```python
from build123d import *

# Parameters (mm, degrees)
SKETCH2_R           = 12.5
SKETCH2_R_2         = 15
BOSS_EXTRUDE1_DEPTH = 5


with BuildPart() as part:
    # Sketch2 → Boss-Extrude1 (new body)
    with BuildSketch(Plane.XY):
        with BuildLine():
            ThreePointArc((0, 25), (-25, 0), (0, -25))
            ThreePointArc((0, -25), (28.284271247, -36.715728753), (40, -65))
            ThreePointArc((40, -65), (55.168868326, -87.985840207), (82.267908001, -83.078145737))
            ThreePointArc((82.267908001, -83.078145737), (117.800748333, 0), (82.267908001, 83.078145737))
            ThreePointArc((82.267908001, 83.078145737), (55.168868326, 87.985840207), (40, 65))
            ThreePointArc((40, 65), (28.284271247, 36.715728753), (0, 25))
        make_face()
        Circle(SKETCH2_R, mode=Mode.SUBTRACT)
        with Locations((65, 65)):
            Circle(SKETCH2_R, mode=Mode.SUBTRACT)
        with Locations((65, -65)):
            Circle(SKETCH2_R_2, mode=Mode.SUBTRACT)
        Polygon((75.334929147, -6.098298085), (75.448745635, 5.901162145), (65.113816488, 11.99946023), (54.665070853, 6.098298085), (54.551254365, -5.901162145), (64.886183512, -11.99946023), align=None, mode=Mode.SUBTRACT)
    extrude(amount=BOSS_EXTRUDE1_DEPTH)


solid = part.part
```
Design review of the part built by this model. Coordinates are the model's own, in mm. A direction names the side the tool comes from. Give positions to 0.01 mm unless a question says otherwise; leave off trailing zeros. Write each loop counter-clockwise with the first axis right and the second up, starting at its lowest first coordinate (ties: lowest second). Pieces come first, ordered by that corner, then holes. Notation, with made-up numbers: (67, 41) -> (87, 41) arc R22 cw to (87, 59) -> close; hole circle Ø7 at (16, -6). An arc over 180 degrees is marked (long way). Answer in a Markdown table with one row per item.
(1) For faces 5 (the cylindrical face through (117.793, -1.3, 2.465)), 6 (the flat face through (70.35, 8.91, 2.46)), list the 3-axis set-ups (+Z, -Z, +X, -X, +Y, -Y) from which the entire face can be reached by the end or side of a thin tool; tool diameter is ignored.
Results:
| item | result |
|---|---|
| face 5 | +Z, -Z, +X |
| face 6 | +Z, -Z |
(2) Mouldability with a two-part tool opening along Y and no side actions: class faces 1 (the cylindrical face through (27.972, -36.406, 2.465)), 2 (the cylindrical face through (28.594, 37.028, 2.465)), 3 (the cylindrical face through (55.79, 73.45, 2.46)), 4 (the flat face through (77, 1, 5)) as +Y half, -Y half, draft (parallel to the pull), parting line (faces both ways), or undercut.
Results:
| item | result |
|---|---|
| face 1 | -Y half |
| face 2 | +Y half |
| face 3 | undercut |
| face 4 | draft |
(3) Consider section B-B (y = 58.5). State the section outline as (x, z) points, then the cut area to 3 significant figures.
Results:
| item | result |
|---|---|
| outline | (39.47, 0) -> (54.32, 0) -> (54.32, 5) -> (39.47, 5) -> close; (75.68, 0) -> (101.79, 0) -> (101.79, 5) -> (75.68, 5) -> close |
| area | 205 mm2 |
(4) Consider section D-D (x = 98). State the section outline as (y, z) points.
Results:
| item | result |
|---|---|
| outline | (-64.48, 0) -> (64.48, 0) -> (64.48, 5) -> (-64.48, 5) -> close |
(5) Clearance check with flat-ended pins moving along their axes: pin 1 (3 mm diameter, centred on x = 92, z = 1, fed in from -Y); pin 2 (20 mm diameter, centred on x = 65, y = 65, fed in from +Z). State where each tip first meets the part, or that it passes through.
Results:
| item | result |
|---|---|
| pin 1 | y = -74.35 |
| pin 2 | through |
(6) Consider section C-C (y = 0). State the section outline as (x, z) points.
Results:
| item | result |
|---|---|
| outline | (-25, 0) -> (-12.5, 0) -> (-12.5, 5) -> (-25, 5) -> close; (12.5, 0) -> (54.61, 0) -> (54.61, 5) -> (12.5, 5) -> close; (75.39, 0) -> (117.8, 0) -> (117.8, 5) -> (75.39, 5) -> close |
(7) Consider section A-A (z = 4.1). State the section outline as (x, y) points.
Results:
| item | result |
|---|---|
| outline | (0, -25) arc R40 cw to (40, -65) arc R25 ccw to (82.27, -83.08) arc R114.89 ccw to (82.27, 83.08) arc R25 ccw to (40, 65) arc R40 cw to (0, 25) arc R25 ccw to start; hole circle Ø25 at (0, 0); hole circle Ø30 at (65, -65); hole circle Ø25 at (65, 65); hole (54.55, -5.9) -> (64.89, -12) -> (75.33, -6.1) -> (75.45, 5.9) -> (65.11, 12) -> (54.67, 6.1) -> close |
(8) To check wall thickness, follow probe 1 along Y at (x, z) = (65, 1.25); probe 2 along X at (y, z) = (-8.5, 2.6); probe 3 along Y at (x, z) = (75, 0.5). State the ranges of each line that lie inside material, in increasing order.
Results:
| item | result |
|---|---|
| probe 1 | -90 to -80, -50 to -11.94, 11.94 to 52.5, 77.5 to 90 |
| probe 2 | -23.51 to -9.17, 9.17 to 58.96, 71.08 to 117.49 |
| probe 3 | -87.91 to -76.18, -53.82 to -6.29, 6.17 to 57.5, 72.5 to 87.91 |
